For this review, take the finished solid that the model builds, in its own axes (mm). A direction names the side the tool comes from. Round coordinates to 2 decimals unless told otherwise and drop trailing zeros. Order: outer loops, then holes, each group sorted by start corner. A loop starts at its lowest first (then second) coordinate and runs counter-clockwise, first axis right, second up. Notation, with made-up numbers: (-14, 41) -> (45, 41) arc R10 ccw to (45, 57) -> close; hole circle Ø8 at (21, 36.25). An arc over 180 degrees is marked (long way). Use a Markdown table: item, result. Add a question column.
1) Draft analysis for pull direction Z (two halves, no side actions). For faces 1 (the face through (-6.436, 4.722, 0.067)), 2 (the face through (10, 6.35, 2)), 3 (the face through (0, 2, 4.762)), 4 (the face through (14.34, 3.22, -0.77)), state which applies: pulls with the +Z half, pulls with the -Z half, needs draft (parallel to the pull), parting line crosses it, or undercut.
2) Wall thickness on line 1 along X through (y, z) = (4, -2) (3 decimals); line 2 along X through (y, z) = (0.75, -0.25) (3 decimals); line 3 along X through (y, z) = (3.5, 1) (3 decimals): over which ranges is each line inside the solid? List them lowest first. Write a range as [from, to].
3) Machinability: for faces 5 (the face through (6.46, 4.72, -0.07)), 6 (the face through (-9.471, 3.219, -0.767)), which of the approach directions +Z, -Z, +X, -X, +Y, -Y give a long, thin tool a straight path to every point of the face, cutting with its end or side? Answer none if there is none.
4) Consider section C-C (y = 0.75). State the section outline as (x, z) points (1 decimal), plus the area to 3 significant figures.
5) Consider section A-A (y = 5.5). State the section outline as (x, z) points (1 decimal), plus the area to 3 significant figures.
6) Consider section B-B (z = 1.25). State the section outline as (x, y) points (3 decimals), plus the area to 3 significant figures.
7) Consider section D-D (x = 12). State the section outline as (y, z) points.
```python
from build123d import *

# Parameters (mm, degrees)
SKETCH1_W                  = 31.75
SKETCH1_H                  = 9.525
BOSS_EXTRUDE1_DEPTH        = 6.35
F_10_CLEARANCE_HOLE1_D     = 5.1054
F_10_CLEARANCE_HOLE1_DEPTH = 19.05
F_10_CLEARANCE_HOLE1_TIP   = 1.533816902
CUT_EXTRUDE1_DEPTH         = 3.302


with BuildPart() as part:
    # Sketch1 → Boss-Extrude1 (new body)
    with BuildSketch(Plane(origin=(0, 0, 0), x_dir=(1, 0, 0), z_dir=(0, 1, 0))):
        Rectangle(SKETCH1_W, SKETCH1_H)
    extrude(amount=BOSS_EXTRUDE1_DEPTH)

    # #10 Clearance Hole1
    with Locations(Plane(origin=(0, 0, 0), x_dir=(-1, 0, 0), z_dir=(0, -1, 0))):
        with Locations((11.90625, 0), (-11.90625, 0)):
            Hole(F_10_CLEARANCE_HOLE1_D / 2, depth=F_10_CLEARANCE_HOLE1_DEPTH)
            with Locations((0, 0, -(F_10_CLEARANCE_HOLE1_DEPTH + F_10_CLEARANCE_HOLE1_TIP / 2))):  # 118° drill point
                Cone(0, F_10_CLEARANCE_HOLE1_D / 2, F_10_CLEARANCE_HOLE1_TIP, mode=Mode.SUBTRACT)

    # Sketch4 → Cut-Extrude1 (cut)
    with BuildSketch(Plane(origin=(0, 6.35, 0), x_dir=(1, 0, 0), z_dir=(0, 1, 0))):
        Polygon((7.287716231, 4.7625), (5.60820174, -4.7625), (-5.60820174, -4.7625), (-7.287716231, 4.7625), align=None)
    extrude(amount=-CUT_EXTRUDE1_DEPTH, mode=Mode.SUBTRACT)


solid = part.part
```
Results list:
| question | item | result |
|---|---|---|
| 1 | face 1 | pulls with the -Z half |
| 1 | face 2 | needs draft |
| 1 | face 3 | pulls with the +Z half |
| 1 | face 4 | undercut |
| 2 | line 1 | [-15.875, -13.493], [-10.32, -6.801], [6.801, 10.32], [13.493, 15.875] |
| 2 | line 2 | [-15.875, -14.447], [-9.366, 9.366], [14.447, 15.875] |
| 2 | line 3 | [-15.875, -14.255], [-9.558, -6.272], [6.272, 9.558], [14.255, 15.875] |
| 3 | face 5 | -Z, +Y |
| 3 | face 6 | +Y, -Y |
| 4 | outline | (-15.9, -4.8) -> (15.9, -4.8) -> (15.9, 4.8) -> (-15.9, 4.8) -> close; hole circle Ø5.1 at (-11.9, 0); hole circle Ø5.1 at (11.9, 0) |
| 4 | area | 261 mm2 |
| 5 | outline | (-15.9, -4.8) -> (-7.3, -4.8) -> (-5.6, 4.8) -> (-15.9, 4.8) -> close; (5.6, 4.8) -> (7.3, -4.8) -> (15.9, -4.8) -> (15.9, 4.8) -> close; hole circle Ø5.1 at (-11.9, 0); hole circle Ø5.1 at (11.9, 0) |
| 5 | area | 139 mm2 |
| 6 | outline | (-15.875, 0) -> (-14.132, 0) -> (-14.132, 6.35) -> (-15.875, 6.35) -> close; (-9.681, 0) -> (9.681, 0) -> (9.681, 6.35) -> (6.228, 6.35) -> (6.228, 3.048) -> (-6.228, 3.048) -> (-6.228, 6.35) -> (-9.681, 6.35) -> close; (14.132, 0) -> (15.875, 0) -> (15.875, 6.35) -> (14.132, 6.35) -> close |
| 6 | area | 104 mm2 |
| 7 | outline | (0, -4.76) -> (6.35, -4.76) -> (6.35, -2.55) -> (0, -2.55) -> close; (0, 2.55) -> (6.35, 2.55) -> (6.35, 4.76) -> (0, 4.76) -> close |
